Model file for the job. Use its own axes, mm. A direction names the side the tool comes from. Give positions to 0.01 mm unless a question says otherwise; leave off trailing zeros. Write each loop counter-clockwise with the first axis right and the second up, starting at its lowest first coordinate (ties: lowest second). Pieces come first, ordered by that corner, then holes. Notation, with made-up numbers: M 54.5,50 L 94.5,50 A28 cw 94.5,69 Z; hole C 32,37.5 d2. An arc over 180 degrees is marked long. Answer as a JSON object with one key per item and string values. Group by question number.
```python
from build123d import *

# Parameters (mm, degrees)
IZIM1_W                     = 170
IZIM1_H                     = 200
Y_KSEKLIK_EKSTR_ZYON1_DEPTH = 20
IZIM2_W                     = 130
IZIM2_H                     = 20
Y_KSEKLIK_EKSTR_ZYON2_DEPTH = 100
RADYUS1_R                   = 20
IZIM3_R                     = 20
KES_EKSTR_ZYON1_DEPTH       = 100
IZIM4_R                     = 20
Y_KSEKLIK_EKSTR_ZYON3_DEPTH = 20
IZIM5_W                     = 170
IZIM5_H                     = 40
IZIM5_H_2                   = 80
KES_EKSTR_ZYON2_DEPTH       = 79


with BuildPart() as part:
    # Çizim1 → Yükseklik-Ekstrüzyon1 (new body)
    with BuildSketch(Plane.XY):
        with Locations((85, 100)):
            Rectangle(IZIM1_W, IZIM1_H)
    extrude(amount=Y_KSEKLIK_EKSTR_ZYON1_DEPTH)

    # Çizim2 → Yükseklik-Ekstrüzyon2 (add)
    with BuildSketch(Plane(origin=(0, 0, 0), x_dir=(-1, 0, 0), z_dir=(0, 0, -1))):
        with Locations((-85, 140)):
            Rectangle(IZIM2_W, IZIM2_H)
    extrude(amount=Y_KSEKLIK_EKSTR_ZYON2_DEPTH)

    # Radyus1
    radyus1_edges = [part.edges().sort_by_distance(p)[0] for p in [
        (150, 140, -100),
        (20, 140, -100),
    ]]
    fillet(radyus1_edges, radius=RADYUS1_R)

    # Çizim3 → Kes-Ekstrüzyon1 (cut)
    with BuildSketch(Plane(origin=(0, 150, 0), x_dir=(1, 0, 0), z_dir=(0, 1, 0))):
        with Locations(Location((85, 50, 0), (0, 0, 180))):
            Circle(IZIM3_R)
    extrude(amount=-KES_EKSTR_ZYON1_DEPTH, mode=Mode.SUBTRACT)

    # Çizim4 → Yükseklik-Ekstrüzyon3 (add)
    with BuildSketch(Plane(origin=(0, 110, 0), x_dir=(-1, 0, 0), z_dir=(0, -1, 0))):
        with BuildLine():
            Line((-20, 0), (-20, 80))
            ThreePointArc((-20, 80), (-25.857864376, 94.142135624), (-40, 100))
            Line((-40, 100), (-130, 100))
            ThreePointArc((-130, 100), (-144.142135624, 94.142135624), (-150, 80))
            Line((-150, 80), (-150, 0))
            Line((-150, 0), (-20, 0))
        make_face()
        with Locations((-85, 50)):
            Circle(IZIM4_R, mode=Mode.SUBTRACT)
    extrude(amount=Y_KSEKLIK_EKSTR_ZYON3_DEPTH)

    # Çizim5 → Kes-Ekstrüzyon2 (cut)
    with BuildSketch(Plane(origin=(0, 0, 0), x_dir=(-1, 0, 0), z_dir=(0, 0, -1))):
        with Locations((-85, 180)):
            Rectangle(IZIM5_W, IZIM5_H)
        with Locations((-85, 40)):
            Rectangle(IZIM5_W, IZIM5_H_2)
    extrude(amount=-KES_EKSTR_ZYON2_DEPTH, mode=Mode.SUBTRACT)


solid = part.part
```
Q1. Slice it at C-C, the plane z = -50. Write the cut outline in (x, y), then the cut area to 3 significant figures.
Q2. Two-plate mould, pull along X, no slides. Class faces 6 (the cylindrical face through (144.297, 140.14, -93.986)), 7 (the flat face through (86, 130, -27)), 8 (the flat face through (0, 119, 10)), 9 (the cylindrical face through (104.98, 140.14, -49.12)): +X half, -X half, draft (parallel to the pull), parting line (faces both ways), or undercut.
Q3. Drop flat-ended pins along their axis: P1, Ø6, axis at y = 101.5, z = -23, coming from the -X side; P2, Ø16, axis at y = 101, z = -45.5, coming from the +X side; P3, Ø1, axis at x = 146, y = 117, coming from the -Z side. Give the stop position or say it passes through.
Q4. Wall check: L1, parallel to Y at x = 95.5, z = -28.5; L2, parallel to X at y = 103, z = -50; L3, parallel to Z at x = 85, y = 98.5. Give the ranges that are in metal, low to high.
Q5. Slice it at B-B, the plane z = -26. Write the cut outline in (x, y).
Q6. Slice it at D-D, the plane y = 101.5. Write the cut outline in (x, z), then the cut area to 3 significant figures.
Q7. 3-axis set-ups, long thin cutter, end or side, ignore diameter. For faces 1 (the flat face through (86, 150, -27)), 2 (the flat face through (150, 140, -39)), 3 (the flat face through (20, 140, -39)), 4 (the flat face through (86, 110, -28)), 5 (the flat face through (86, 90, -28)): which of +Z, -Z, +X, -X, +Y, -Y reach the whole face in a straight line?
Q8. Slice it at A-A, the plane x = 85. Write the cut outline in (y, z).
Solved:
{
 "1": {"outline": "M 20,90 L 65,90 L 65,110 L 20,110 Z; M 20,130 L 65,130 L 65,150 L 20,150 Z; M 105,90 L 150,90 L 150,110 L 105,110 Z; M 105,130 L 150,130 L 150,150 L 105,150 Z", "area": "3,600 mm²"},
 "2": {"face 6": "+X half", "face 7": "draft", "face 8": "-X half", "face 9": "undercut"},
 "3": {"P1": "stops at x = 20", "P2": "stops at x = 150", "P3": "stops at z = 0"},
 "4": {"L1": "y = 90 to 110, 130 to 150", "L2": "x = 20 to 65, 105 to 150", "L3": "z = -100 to -70, -30 to 20"},
 "5": {"outline": "M 20,90 L 150,90 L 150,110 L 20,110 Z; M 20,130 L 150,130 L 150,150 L 20,150 Z"},
 "6": {"outline": "M 0,0 L 20,0 L 20,-80 A20 ccw 40,-100 L 130,-100 A20 ccw 150,-80 L 150,0 L 170,0 L 170,20 L 0,20 Z; hole C 85,-50 d40", "area": "15,000 mm²"},
 "7": {"face 1": "-Z, +X, -X, +Y", "face 2": "-Z, +X, +Y, -Y", "face 3": "-Z, -X, +Y, -Y", "face 4": "-Z, +X, -X", "face 5": "-Z, +X, -X, -Y"},
 "8": {"outline": "M 80,0 L 90,0 L 90,-30 L 110,-30 L 110,0 L 130,0 L 130,-30 L 150,-30 L 150,0 L 160,0 L 160,20 L 80,20 Z; M 90,-100 L 110,-100 L 110,-70 L 90,-70 Z; M 130,-100 L 150,-100 L 150,-70 L 130,-70 Z"}
}
